Read the model definition and answer for the solid it produces. Units are mm, in the model's axes. Face numbers are marked on the shaded views. A direction names the side the tool comes from. Coordinates: 2 decimals unless noted, no trailing zeros. Order: outer loops, then holes, each group sorted by start corner. A loop starts at its lowest first (then second) coordinate and runs counter-clockwise, first axis right, second up. Notation, with made-up numbers: M 12.25,42 L 33.25,42 A24 cw 33.25,66 Z; hole C -8.5,76.25 d11. An arc over 180 degrees is marked long. Use a Markdown table: item, result. Add a question column.
1) Find the intervals of material crossed by probe 1 along Z at (x, y) = (4.5, -4.5); probe 2 along X at (y, z) = (-1.5, 4.35); probe 3 along Z at (x, y) = (0, 1), in increasing order. Write a range as [from, to].
2) For the marked faces 5, 6, 7, 8 and 9, determine the directions among +Z, -Z, +X, -X, +Y, -Y from which every point of the face is accessible in a straight line to the end or side of a thin tool.
3) Each of these flat-tipped pins is pushed along its axis until it touches: pin 1 Ø0.9 at (y, z) = (-2, 4.5) entering from -X; pin 2 Ø1.4 at (y, z) = (-2.5, 5.5) entering from +X; pin 3 Ø2 at (y, z) = (1.5, 5) entering from -X. Where does it stop, or does it pass through?
4) Find section D-D on x = -0.75. Write down the section's boundary in (y, z).
5) The mould has two halves that part along Z. Classify the marked faces 1, 2, 3 and 4: released by +Z, released by -Z, zero draft, split by the parting line, or undercut.
6) Find section C-C on x = -5. Write down the section's boundary in (y, z).
7) Find section A-A on y = -1. Write down the section's boundary in (x, z).
8) Find section B-B on z = 3.15. Write down the section's boundary in (x, y).
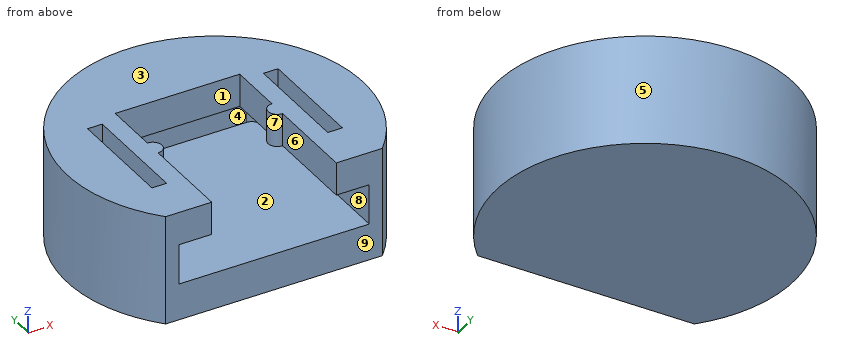
from build123d import *

# Parameters (mm, degrees)
BOSS_EXTRUDE1_DEPTH = 6
SKETCH2_W           = 6.8
SKETCH2_H           = 9
CUT_EXTRUDE1_DEPTH  = 4
SKETCH3_W           = 10.4
SKETCH3_H           = 10.6
CUT_EXTRUDE2_DEPTH  = 2.2
SKETCH4_W           = 0.8
SKETCH4_H           = 6
CUT_EXTRUDE3_DEPTH  = 2.2
SKETCH5_R           = 0.5
BOSS_EXTRUDE2_DEPTH = 1.8
FILLET1_R           = 0.5


with BuildPart() as part:
    # Sketch1 → Boss-Extrude1 (new body)
    with BuildSketch(Plane.XY):
        with BuildLine():
            Line((5.916079783, -5.5), (-5.916079783, -5.5))
            ThreePointArc((-5.916079783, -5.5), (0, 8.077747211), (5.916079783, -5.5))
        make_face()
    extrude(amount=BOSS_EXTRUDE1_DEPTH)

    # Sketch2 → Cut-Extrude1 (cut)
    with BuildSketch(Plane.XY.offset(6)):
        with Locations((0, -1)):
            Rectangle(SKETCH2_W, SKETCH2_H)
    extrude(amount=-CUT_EXTRUDE1_DEPTH, mode=Mode.SUBTRACT)

    # Sketch3 → Cut-Extrude2 (cut)
    with BuildSketch(Plane.XY.offset(2)):
        with Locations((0, -0.2)):
            Rectangle(SKETCH3_W, SKETCH3_H)
    extrude(amount=CUT_EXTRUDE2_DEPTH, mode=Mode.SUBTRACT)

    # Sketch4 → Cut-Extrude3 (cut)
    with BuildSketch(Plane.XY.offset(6)):
        with Locations((-4.8, 0)):
            Rectangle(SKETCH4_W, SKETCH4_H)
        with Locations((4.8, 0)):
            Rectangle(SKETCH4_W, SKETCH4_H)
    extrude(amount=-CUT_EXTRUDE3_DEPTH, mode=Mode.SUBTRACT)

    # Sketch5 → Boss-Extrude2 (add)
    with BuildSketch(Plane.XY.offset(6)):
        with Locations((-3.4, 0)):
            Circle(SKETCH5_R)
        with Locations((3.4, 0)):
            Circle(SKETCH5_R)
    extrude(amount=-BOSS_EXTRUDE2_DEPTH)

    # Fillet1
    fillet1_edges = [part.edges().sort_by_distance(p)[0] for p in [
        (-5.2, 5.1, 3.1),
        (5.2, 5.1, 3.1),
    ]]
    fillet(fillet1_edges, radius=FILLET1_R)


solid = part.part
Check result:
| question | item | result |
|---|---|---|
| 1 | probe 1 | z = [0, 2], [4.2, 6] |
| 1 | probe 2 | x = [-7.94, -5.2], [-4.4, -3.4], [3.4, 4.4], [5.2, 7.94] |
| 1 | probe 3 | z = [0, 2] |
| 2 | face 5 | +Z, -Z |
| 2 | face 6 | +Z, -Y |
| 2 | face 7 | +Z |
| 2 | face 8 | none |
| 2 | face 9 | +Z, -Z, +X, -X, -Y |
| 3 | pin 1 | stops at x = -7.93 |
| 3 | pin 2 | stops at x = 7.87 |
| 3 | pin 3 | stops at x = -8.06 |
| 4 | outline | M -5.5,0 L 8.04,0 L 8.04,6 L 3.5,6 L 3.5,4.2 L 5.1,4.2 L 5.1,2 L -5.5,2 Z |
| 5 | face 1 | zero draft |
| 5 | face 2 | undercut |
| 5 | face 3 | released by +Z |
| 5 | face 4 | undercut |
| 6 | outline | M -5.5,0 L 6.34,0 L 6.34,6 L 3,6 L 3,4.2 L 5,4.2 L 5,2 L -5.5,2 Z; M -5.5,4.2 L -3,4.2 L -3,6 L -5.5,6 Z |
| 7 | outline | M -8.02,0 L 8.02,0 L 8.02,6 L 5.2,6 L 5.2,2 L -5.2,2 L -5.2,6 L -8.02,6 Z; M -4.4,4.2 L -3.4,4.2 L -3.4,6 L -4.4,6 Z; M 3.4,4.2 L 4.4,4.2 L 4.4,6 L 3.4,6 Z |
| 8 | outline | M -5.92,-5.5 L -5.2,-5.5 L -5.2,4.6 A0.5 cw -4.7,5.1 L 4.7,5.1 A0.5 cw 5.2,4.6 L 5.2,-5.5 L 5.92,-5.5 A8.08 ccw long Z |
